Read the model definition and answer for the solid it produces. Units are mm, in the model's axes. Face numbers are marked on the shaded views. A direction names the side the tool comes from. Give positions to 0.01 mm unless a question says otherwise; leave off trailing zeros. Loops run counter-clockwise (first coordinate to the right, second up) from the corner with the lowest first, then second, coordinate; pieces in that order, holes last.
(1) Determine the mould class of the marked faces 1, 2 and 3 for opening direction X: pulls with the +X half, pulls with the -X half, needs draft (parallel to the pull), parting line crosses it, or undercut.
(2) Find section B-B, the plane x = 28. Write down the section's boundary in (y, z), then the cut area to 3 significant figures.
(3) Which of the six approach directions +Z, -Z, +X, -X, +Y, -Y give full straight-line access (tool end or side, diameter ignored) to the marked faces 4, 5, 6, 7 and 8?
(4) Find section D-D, the plane y = 6. Write down the section's boundary in (x, z), then the cut area to 3 significant figures.
(5) Each of these flat-tipped pins is pushed along its axis until it touches: P1, Ø6, axis at y = -16.5, z = -1, coming from the +X side; P2, Ø11, axis at x = 9.5, y = -7, coming from the +Z side; P3, Ø1, axis at x = -20, z = 5.5, coming from the +Y side. Where does it stop, or does it pass through?
(6) Find section A-A, the plane y = -1.5. Write down the section's boundary in (x, z).
(7) Find section C-C, the plane z = 3. State how many separate pieces and enclosed holes the cut face has, then the cut area to 3 significant figures.
(8) Straight lines are drawn through the part: probe 1 along X at (y, z) = (-12, -9.5); probe 2 along Z at (x, y) = (-27.25, -12); probe 3 along Z at (x, y) = (-14, 9). For each, find the intervals that lie inside material, in ascending order.
```python
from build123d import *

# Parameters (mm, degrees)
F1_DEPTH = 16
F2_DEPTH = 4
F3_DEPTH = 10
F4_W     = 10
F4_H     = 20
F5_DEPTH = 22
F6_R     = 6
F7_DEPTH = 75.0009999306
F8_R     = 1.5


# Not quite as in the source:
# - ends of sketch curves that miss each other by under 0.0002 mm in the source are joined


with BuildPart() as f1:
    # F0 (on Top) → F1 (new body, symmetric)
    with BuildSketch(Plane.XY):
        Polygon((14.1706688348, 5), (5.1815587922, 5), (-30.8302634659, 5), (-30.8302634659, 0), (14.1933665337, 0), align=None)
        with BuildLine():
            ThreePointArc((9.1762328499, 9.2063472144), (8.0820233117, 6.2454935885), (5.1815587922, 5))
            Line((5.1815587922, 5), (14.1706688348, 5))
            ThreePointArc((14.1706688348, 5), (15.2379483, 8.3057115079), (18.4888007758, 9.5299550339))
            ThreePointArc((18.4888007758, 9.5299550339), (35.6997870029, 10.0097302467), (44.1697364647, 25))
            Line((44.1697364647, 25), (39.1697364647, 25))
            ThreePointArc((39.1697364647, 25), (26.6697364647, 12.5), (14.1697364647, 25))
            Line((14.1697364647, 25), (9.169736973, 25))
            Line((9.169736973, 25), (9.1697442854, 24.9834553538))
            Line((9.1697442854, 24.9834553538), (9.1762328499, 9.2063472144))
        make_face()
        with BuildLine():
            Line((14.1706688348, 25), (14.1697364647, 25))
            ThreePointArc((14.1697364647, 25), (26.6697364647, 12.5), (39.1697364647, 25))
            Line((39.1697364647, 25), (37.1697364647, 25))
            ThreePointArc((37.1697364647, 25), (26.6697364647, 14.5), (16.1697364647, 25))
            Line((16.1697364647, 25), (14.1706688348, 25))
        make_face()
    extrude(amount=F1_DEPTH, both=True)

    # F0 (on Top) → F2 (join, symmetric)
    with BuildSketch(Plane.XY):
        with BuildLine():
            Line((-30.8302634659, 5), (5.1815587922, 5))
            ThreePointArc((5.1815587922, 5), (8.0820233117, 6.2454935885), (9.1762328499, 9.2063472144))
            Line((9.1762328499, 9.2063472144), (9.1697442854, 24.9834553538))
            Line((9.1697442854, 24.9834553538), (9.1697374812, 25.0000000002))
            Line((9.1697374812, 25.0000000002), (9.168883179, 25))
            Line((9.168883179, 25), (-30.8302634659, 5))
        make_face()
    extrude(amount=F2_DEPTH, both=True)

    # F0 (on Top) → F3 (cut, symmetric)
    with BuildSketch(Plane.XY):
        with BuildLine():
            Line((14.1706688348, 25), (14.1697364647, 25))
            ThreePointArc((14.1697364647, 25), (26.6697364647, 12.5), (39.1697364647, 25))
            Line((39.1697364647, 25), (37.1697364647, 25))
            ThreePointArc((37.1697364647, 25), (26.6697364647, 14.5), (16.1697364647, 25))
            Line((16.1697364647, 25), (14.1706688348, 25))
        make_face()
    extrude(amount=F3_DEPTH, both=True, mode=Mode.SUBTRACT)

    # F4 (on face) → F5 (join)
    with BuildSketch(Plane.XZ):
        with Locations((9.1933665337, 0)):
            Rectangle(F4_W, F4_H)
        Polygon((-20.8302634659, 10), (-30.8302634659, 10), (-30.8302634659, 0), (-30.8302634659, -10), (-20.8302634659, -10), align=None)
    extrude(amount=F5_DEPTH)

    # F6 (on face) → F7 (cut, through all)
    with BuildSketch(Plane(origin=(-30.8302634659, 0, 0), x_dir=(0, -1, 0), z_dir=(-1, 0, 0))):
        with BuildLine():
            Line((22, 10), (12, 10))
            ThreePointArc((12, 10), (19.0710677836, 7.0710678402), (22, 8.01e-08))
            Line((22, 8.01e-08), (22, 10))
        make_face()
        with BuildLine():
            Line((22, -10), (22, 8.01e-08))
            ThreePointArc((22, 8.01e-08), (19.0710678402, -7.0710677836), (12, -10))
            Line((12, -10), (22, -10))
        make_face()
        with Locations((12, 0)):
            Circle(F6_R)
    extrude(amount=-F7_DEPTH, mode=Mode.SUBTRACT)

    # F8
    f8_edges = [f1.edges().sort_by_distance(p)[0] for p in [
        (-30.830263, -6, 0),
        (-20.830263, -6, 0),
        (14.193367, -6, 0),
        (4.193367, -6, 0),
    ]]
    fillet(f8_edges, radius=F8_R)


solid = f1.part
```
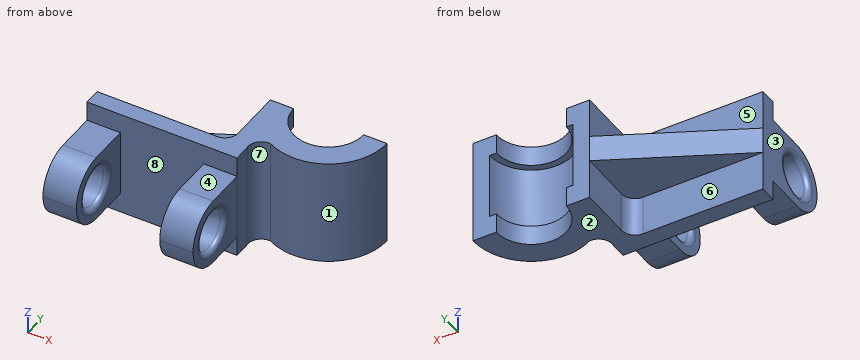
Entries:
1. face 1: undercut
1. face 2: needs draft
1. face 3: pulls with the -X half
2. outline: (7.55, -16) - (14.58, -16) - (14.58, -10) - (12.57, -10) - (12.57, 10) - (14.58, 10) - (14.58, 16) - (7.55, 16) - close
2. area: 185 mm2
3. face 4: +Z, +X, -X, -Y
3. face 5: +Z, -X, +Y
3. face 6: -Z, -X, +Y
3. face 7: +Z, -Z
3. face 8: -Y
4. outline: (-28.83, -4) - (7.83, -4) - (7.83, -16) - (14.16, -16) - (14.16, 16) - (7.83, 16) - (7.83, 4) - (-28.83, 4) - close
4. area: 496 mm2
5. P1: stops at x = 14.19
5. P2: stops at z = 10
5. P3: stops at y = 5
6. outline: (-30.83, -10) - (-20.83, -10) - (-20.83, 10) - (-30.83, 10) - close; (4.19, -10) - (14.19, -10) - (14.19, 10) - (4.19, 10) - close
7. separate pieces: 3
7. enclosed holes: 0
7. area: 1,150 mm2
8. probe 1: x = -30.83 to -20.83, 4.19 to 14.19
8. probe 2: z = -10 to -6, 6 to 10
8. probe 3: z = -4 to 4
